Geometry: final body of the model. Coordinates: model frame, mm. A direction names the side the tool comes from. Give positions to 0.01 mm unless a question says otherwise; leave off trailing zeros. Write each loop counter-clockwise with the first axis right and the second up, starting at its lowest first coordinate (ties: lowest second). Pieces come first, ordered by that corner, then holes. Notation, with made-up numbers: M 31,65.25 L 89,65.25 A30 ccw 89,87.25 Z; hole C 34.25,26.5 d3. An arc over 180 degrees is marked long. Use a Markdown table: item, result. Add a question column.
(1) Cut plane C-C (x = 8). Output: boundary loops of the cut face in (y, z).
(2) Cut plane A-A (z = 0). Output: boundary loops of the cut face in (x, y).
(3) Draft query along Y for faces 4 (the flat face through (0, 4, 0)), 5 (the flat face through (-1.5, 0, 0)), 6 (the flat face through (-3, 0.8, 0)), 7 (the cylindrical face through (-2.03, -2.17, 9.76)). Return one class per face: released by +Y, released by -Y, zero draft, split by the parting line, or undercut.
(4) Pin query (flat end, axial travel): pin 1 Ø1.2 at (x, z) = (-3, -4.5) entering from +Y; pin 2 Ø4 at (x, y) = (8, 2.5) entering from +Z; pin 3 Ø0.5 at (y, z) = (0, -4.5) entering from -X; pin 4 Ø8 at (x, y) = (8.5, 7.5) entering from -Z. Return the tip coordinate at first contact, or that it passes through.
(5) Cut plane B-B (y = 0). Output: boundary loops of the cut face in (x, z), plus the area to 3 significant figures.
(6) Cut plane D-D (z = -7.5). Output: boundary loops of the cut face in (x, y).
(7) Material intervals for L1, parallel to X at y = -6.5, z = 2.75; L2, parallel to Y at x = -3, z = -7.75; L3, parallel to Y at x = 2, z = 1.5, sorted ascending.
(8) Reachability of faces 1 (the flat face through (-4, -4, 0)), 2 (the flat face through (-3, -0.8, 0)), 3 (the cylindrical face through (5, -3, 0)) from +Z, -Z, +X, -X, +Y, -Y: full face, straight path, thin tool, end or side. Return the list, or none.
Autodesk Inventor part; units mm, degrees
ref_plane "Work Plane1" through (30.1625, 0, 0) normal (0, 0, -1) x (1, 0, 0)
ref_plane "YZ Plane" through (0, 0, 0) normal (1, 0, 0) x (0, 1, 0)
ref_plane "XZ Plane" through (0, 0, 0) normal (0, 1, 0) x (-1, 0, 0)
sketch "Sketch1" plane through (0, 0, 0) normal (0, 0, 1) x (1, 0, 0)
  line L0 (-4, 0) -> (10, 0)
  line L1 (10, 0) -> (10, 3)
  line L2 (10, 3) -> (1, 3)
  line L3 (1, 3) -> (0.3865, 3.1)
  line L4 (0.3865, 3.1) -> (0.25, 3.1)
  line L5 (0, 3.35) -> (0, 10)
  line L6 (-6.8, 0) -> (12.8, 0)
  line L7 (0, -2) -> (0, 12)
  line L8 (-4, 0) -> (-4, 9.9999)
  line L9 (0, 10) -> (-4, 9.9999)
  arc A0 (0, 3.35) -> (0.25, 3.1) centre (0.25, 3.35) ccw
  point P0 (0, 3.1)
  dimension "d0" = 10
  dimension "d1" = 9
  dimension "d2" = 0.6135
  dimension "d3" = 4
  dimension "d4" = 6
  dimension "d5" = 6.2
  dimension "d9" = 20
  dimension "d10" = 0.001
  dimension "d40" = 0.25
revolve "Body" add sketch "Sketch1" angle 360 about axis through (-4, 0, 0) along (1, 0, 0)
sketch "Sketch2" plane through (-4, 0, 0) normal (-1, 0, 0) x (0, 0, 1)
  circle A0 centre (0, 0) radius 10
  line L0 (0, 0) -> (0, 9.9999)
  line L1 (-10, 0.8) -> (10, 0.8)
  line L2 (10, 0.8) -> (10, -0.8)
  line L3 (10, -0.8) -> (-10, -0.8)
  line L4 (-10, -0.8) -> (-10, 0.8)
  line L5 (-10, 0) -> (10, 0) construction
  line L6 (0, 0.8) -> (0, -0.8) construction
  dimension "d11" = 1.6
  dimension "d12" = 20
fillet "Fillet1" radius 0.0001 1 edges at (-4, -9.9999, 0)
extrude "Slot" cut sketch "Sketch2" against normal blind 2.5 contours A0 L3 L1 | L2 L3 A0 | A0 L1 L2 | L3 L4 A0 | A0 L4 L1
thread "Thread"
sketch "Sketch3" plane through (0, 0, 0) normal (0, 0, 1) x (1, 0, 0)
  line L0 (10, 0) -> (10, 3)
  line L1 (10, 3) -> (1, 3)
  line L2 (-4, 0) -> (10, 0)
  line L3 (10, -3) -> (10, 3)
  line L4 (1, -3) -> (10, -3)
  arc A0 (8.7394, -3) -> (8.7394, 3) centre (5.8, 0) ccw
  dimension "d41" = 8.4
revolve "Fillet2" cut sketch "Sketch3" angle 360 about axis through (-4, 0, 0) along (1, 0, 0) contours A0 L1 L0
ref_plane "Work Plane1" through (30.1625, 0, 0) normal (0, 0, -1) x (1, 0, 0)
equation "\"d11\" = SBR"
equation "\"d12\" = KOD"
equation "\"d13\" = RR"
equation "\"d16\" = STI"
equation "\"d14\" = GEL"
equation "\"d0\" = NLG"
equation "\"d1\" = GEL"
equation "\"d2\" = GAL"
equation "\"d3\" = KOH"
equation "\"d4\" = GD"
equation "\"d5\" = BDM"
equation "\"d9\" = KOD"
equation "\"d10\" = KEWI"
equation "\"d40\" = R"
equation "\"d41\" = RE"
equation "\"GD\" = NND"
equation "\"NLG\" = 10"
equation "\"GEL\" = 9"
equation "\"KOD\" = 20"
equation "\"KOH\" = 4"
equation "\"GAL\" = 0.61345 * PTC"
equation "\"BDM\" = 6.2"
equation "\"RR\" = 0.0001"
equation "\"SBR\" = 1.6"
equation "\"STI\" = 2.5"
equation "\"KEWI\" = 0.001deg"
equation "\"R\" = 0.25"
equation "\"RE\" = 8.4"
equation "\"GUL\" = 0.61345 * PTC"
equation "\"SPD\" = NND - 1.2269 * PTC"
equation "\"PTC\" = 1"
equation "\"THREADDIA\" = 6"
equation "\"TOA\" = 30deg"
equation "\"FAWI\" = 45"
equation "\"NND\" = 6"
equation "\"GD1\" = THREADDIA - 1.2269 * PTC"
properties part number "Screw GB 833 M6 x 10" material "Steel, Mild"
Answer list:
| question | item | result |
|---|---|---|
| 1 | outline | C 0,0 d6 |
| 2 | outline | M -4,-10 L 0,-10 L 0,-3.35 A0.25 cw 0.25,-3.1 L 0.39,-3.1 L 1,-3 L 8.74,-3 A4.2 ccw 8.74,3 L 1,3 L 0.39,3.1 L 0.25,3.1 A0.25 cw 0,3.35 L 0,10 L -4,10 L -4,0.8 L -1.5,0.8 L -1.5,-0.8 L -4,-0.8 Z |
| 3 | face 4 | zero draft |
| 3 | face 5 | undercut |
| 3 | face 6 | undercut |
| 3 | face 7 | split by the parting line |
| 4 | pin 1 | y = 9.21 |
| 4 | pin 2 | z = 2.96 |
| 4 | pin 3 | x = -1.5 |
| 4 | pin 4 | through |
| 5 | outline | M -1.5,-10 L 0,-10 L 0,-3.35 A0.25 cw 0.25,-3.1 L 0.39,-3.1 L 1,-3 L 8.74,-3 A4.2 ccw 8.74,3 L 1,3 L 0.39,3.1 L 0.25,3.1 A0.25 cw 0,3.35 L 0,10 L -1.5,10 Z |
| 5 | area | 87.8 mm² |
| 6 | outline | M -4,-6.61 L 0,-6.61 L 0,6.61 L -4,6.61 L -4,0.8 L -1.5,0.8 L -1.5,-0.8 L -4,-0.8 Z |
| 7 | L1 | -4 to 0 |
| 7 | L2 | -6.32 to -0.8, 0.8 to 6.32 |
| 7 | L3 | -2.6 to 2.6 |
| 8 | face 1 | +Z, -Z, -X, +Y, -Y |
| 8 | face 2 | +Z, -Z, -X |
| 8 | face 3 | +X |
